Can you work these out from the drawing? Everything is in mm from the part's minimum corner. Coordinates: 2 decimals unless noted, no trailing zeros. Loops run counter-clockwise (first coordinate to the right, second up) from the corner with the lowest first, then second, coordinate; pieces in that order, holes last. Notation, with made-up numbers: M 70,78.25 L 94,78.25 A28 cw 94,110.25 Z; hole C -37,84.25 d10. An arc over 180 degrees is marked long. Write each question's results on one line, items separated by ' | '.
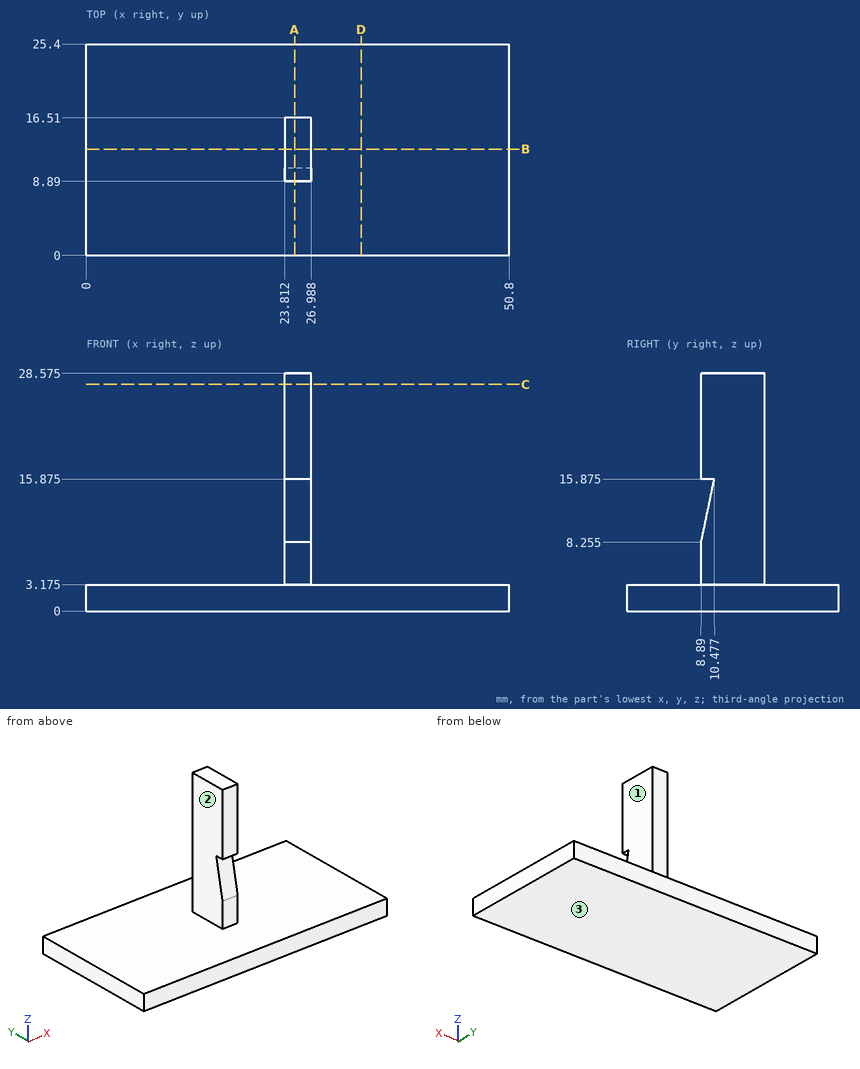
(1) Imagine slicing it at A-A, the plane x = 25. List the corners of the cut face in (y, z) for me (1 decimal).
Reported:
outline: M 0,0 L 25.4,0 L 25.4,3.2 L 16.5,3.2 L 16.5,28.6 L 8.9,28.6 L 8.9,15.9 L 10.5,15.9 L 8.9,8.3 L 8.9,3.2 L 0,3.2 Z
(2) Imagine slicing it at C-C, the plane z = 27.25. List the corners of the cut face in (x, y) for me.
Reported:
outline: M 23.81,8.89 L 26.99,8.89 L 26.99,16.51 L 23.81,16.51 Z
(3) If we mould it in two halves opening along X, with no side actions, what happens to the marked faces 1, 2 and 3? For each: released by +X, released by -X, zero draft, split by the parting line, or undercut.
Reported:
face 1: released by +X | face 2: released by -X | face 3: zero draft
(4) Will these pins go through, and if not, where does the flat tip stop? P1, Ø1, axis at y = 12, z = 17.5, coming from the +X side; P2, Ø4, axis at x = 20, y = 15, coming from the +Z side (1 decimal); P3, Ø4, axis at x = 10, z = 3.5, coming from the -Y side; P4, Ø4, axis at y = 13.5, z = 17, coming from the -X side.
Reported:
P1: stops at x = 26.99 | P2: stops at z = 3.2 | P3: stops at y = 0 | P4: stops at x = 23.81
(5) Please list where these lines run through material, in increasing order: probe 1 along Z at (x, y) = (42.5, 12) (1 decimal); probe 2 along X at (y, z) = (14, 15.75). Write a range as from..to.
Reported:
probe 1: z = 0..3.2 | probe 2: x = 23.81..26.99
(6) Imagine slicing it at D-D, the plane x = 33. List the corners of the cut face in (y, z) for me (1 decimal).
Reported:
outline: M 0,0 L 25.4,0 L 25.4,3.2 L 0,3.2 Z
(7) Imagine slicing it at B-B, the plane y = 12.75. List the corners of the cut face in (x, z) for me (1 decimal).
Reported:
outline: M 0,0 L 50.8,0 L 50.8,3.2 L 27,3.2 L 27,28.6 L 23.8,28.6 L 23.8,3.2 L 0,3.2 Z
